The model under review builds one solid part; all positions refer to its coordinate system, in mm. A direction names the side the tool comes from. Coordinates: 2 decimals unless noted, no trailing zeros.
1) Machinability: for faces 1 (the flat face through (35, 0, 0)), 2 (the flat face through (43, 0, -14)), 3 (the conical face through (-40.1, 0.7, -13.8)), 4 (the flat face through (-39, 0, 10.75)), 5 (the flat face through (22, 0, -3.75)), which of the approach directions +Z, -Z, +X, -X, +Y, -Y give a long, thin tool a straight path to every point of the face, cutting with its end or side? Answer none if there is none.
2) Mouldability with a two-part tool opening along Z and no side actions: class faces 6 (the conical face through (-40.1, 0.7, 13.7)), 7 (the flat face through (-1, -1.5, 0)), 8 (the cylindrical face through (-42.61, -0.51, 14.21)) as released by +Z, released by -Z, zero draft, split by the parting line, or undercut.
3) Add section A-A, the plane y = -0.75. Give the number of separate pieces and of enclosed holes in the cut face, then the cut area to 3 significant figures.
4) For P1, Ø1.5, axis at y = -0.5, z = 9.5, coming from the -X side; P2, Ø0.9, axis at y = -0.5, z = -7.5, coming from the +X side, all flat-tipped, find the tip position at first contact; note any pin that passes through.
5) For line 1 (Z direction, x = 41.5, y = -0.8); line 2 (X direction, y = 0.8, z = -6); line 3 (Z direction, x = 37.5, y = 0.65), list the stretches that pass through material, from the lowest coordinate up.
from build123d import *

# Parameters (mm, degrees)
SKETCH1_W                                           = 86
SKETCH1_H                                           = 33.5
SKETCH1_W_2                                         = 20
SKETCH1_H_2                                         = 7
BOSS_EXTRUDE1_DEPTH                                 = 1.5
CSK_FOR_M3_COUNTERSUNK_FLAT_HEAD_SCREW1_D           = 3.4
CSK_FOR_M3_COUNTERSUNK_FLAT_HEAD_SCREW1_DEPTH       = 6
CSK_FOR_M3_COUNTERSUNK_FLAT_HEAD_SCREW1_CSINK_D     = 6.3
CSK_FOR_M3_COUNTERSUNK_FLAT_HEAD_SCREW1_CSINK_ANGLE = 90
CSK_FOR_M3_COUNTERSUNK_FLAT_HEAD_SCREW1_TIP         = 1.021463052
TAP_DRILL_FOR_M3_TAP1_D                             = 2.5
SKETCH13_W                                          = 3.5
SKETCH13_H                                          = 18
CUT_EXTRUDE3_DEPTH                                  = 48.943325917
CSK_FOR_M2_COUNTERSUNK_FLAT_HEAD_SCREW3_D           = 2.4
CSK_FOR_M2_COUNTERSUNK_FLAT_HEAD_SCREW3_DEPTH       = 4
CSK_FOR_M2_COUNTERSUNK_FLAT_HEAD_SCREW3_CSINK_D     = 4.4
CSK_FOR_M2_COUNTERSUNK_FLAT_HEAD_SCREW3_CSINK_ANGLE = 90
CSK_FOR_M2_COUNTERSUNK_FLAT_HEAD_SCREW3_TIP         = 0.721032743
SKETCH21_W                                          = 8
SKETCH21_H                                          = 21.5
CUT_EXTRUDE4_DEPTH                                  = 47.244594279
FILLET2_R                                           = 1


with BuildPart() as part:
    # Sketch1 → Boss-Extrude1 (new, symmetric)
    with BuildSketch(Plane(origin=(0, 0, 0), x_dir=(1, 0, 0), z_dir=(0, 1, 0))):
        Rectangle(SKETCH1_W, SKETCH1_H)
        with Locations((22.5, 7.25)):
            Rectangle(SKETCH1_W_2, SKETCH1_H_2, mode=Mode.SUBTRACT)
    extrude(amount=BOSS_EXTRUDE1_DEPTH, both=True)

    # CSK for M3 Countersunk Flat Head Screw1
    with Locations(Plane(origin=(0, 1.5, 0), x_dir=(1, 0, 0), z_dir=(0, 1, 0))):
        with Locations((-32, 8.93052757), (-32, -1.06947243)):
            CounterSinkHole(CSK_FOR_M3_COUNTERSUNK_FLAT_HEAD_SCREW1_D / 2, CSK_FOR_M3_COUNTERSUNK_FLAT_HEAD_SCREW1_CSINK_D / 2, depth=CSK_FOR_M3_COUNTERSUNK_FLAT_HEAD_SCREW1_DEPTH, counter_sink_angle=CSK_FOR_M3_COUNTERSUNK_FLAT_HEAD_SCREW1_CSINK_ANGLE)
            with Locations((0, 0, -(CSK_FOR_M3_COUNTERSUNK_FLAT_HEAD_SCREW1_DEPTH + CSK_FOR_M3_COUNTERSUNK_FLAT_HEAD_SCREW1_TIP / 2))):  # 118° drill point
                Cone(0, CSK_FOR_M3_COUNTERSUNK_FLAT_HEAD_SCREW1_D / 2, CSK_FOR_M3_COUNTERSUNK_FLAT_HEAD_SCREW1_TIP, mode=Mode.SUBTRACT)

    # Tap Drill for M3 Tap1 (through all)
    with Locations(Plane(origin=(0, 1.5, 0), x_dir=(1, 0, 0), z_dir=(0, 1, 0))):
        with Locations((-35, 12.75), (-35, -12.75), (35, -12.75), (35, 12.75)):
            Hole(TAP_DRILL_FOR_M3_TAP1_D / 2)

    # Sketch13 → Cut-Extrude3 (cut, through all)
    with BuildSketch(Plane.XZ.offset(11.5)):
        with Locations((-38.25, -0.25)):
            Rectangle(SKETCH13_W, SKETCH13_H)
    extrude(amount=-CUT_EXTRUDE3_DEPTH, mode=Mode.SUBTRACT)

    # CSK for M2 Countersunk Flat Head Screw3
    with Locations(Plane(origin=(0, 1.5, 0), x_dir=(1, 0, 0), z_dir=(0, 1, 0))):
        with Locations((-41.5, -13.75), (-41.5, 13.75), (41.5, 13.75), (41.5, -13.75)):
            CounterSinkHole(CSK_FOR_M2_COUNTERSUNK_FLAT_HEAD_SCREW3_D / 2, CSK_FOR_M2_COUNTERSUNK_FLAT_HEAD_SCREW3_CSINK_D / 2, depth=CSK_FOR_M2_COUNTERSUNK_FLAT_HEAD_SCREW3_DEPTH, counter_sink_angle=CSK_FOR_M2_COUNTERSUNK_FLAT_HEAD_SCREW3_CSINK_ANGLE)
            with Locations((0, 0, -(CSK_FOR_M2_COUNTERSUNK_FLAT_HEAD_SCREW3_DEPTH + CSK_FOR_M2_COUNTERSUNK_FLAT_HEAD_SCREW3_TIP / 2))):  # 118° drill point
                Cone(0, CSK_FOR_M2_COUNTERSUNK_FLAT_HEAD_SCREW3_D / 2, CSK_FOR_M2_COUNTERSUNK_FLAT_HEAD_SCREW3_TIP, mode=Mode.SUBTRACT)

    # Sketch21 → Cut-Extrude4 (cut, through all)
    with BuildSketch(Plane(origin=(0, 1.5, 0), x_dir=(1, 0, 0), z_dir=(0, 1, 0))):
        with Locations((-39, 0)):
            Rectangle(SKETCH21_W, SKETCH21_H)
        with Locations((39, 0)):
            Rectangle(SKETCH21_W, SKETCH21_H)
    extrude(amount=-CUT_EXTRUDE4_DEPTH, mode=Mode.SUBTRACT)

    # Fillet2
    fillet2_edges = [part.edges().sort_by_distance(p)[0] for p in [
        (35, 0, 10.75),
        (43, 0, 10.75),
        (43, 0, -10.75),
        (35, 0, -10.75),
        (-43, 0, 10.75),
        (-35, 0, 10.75),
        (-43, 0, -10.75),
        (-35, 0, -10.75),
        (12.5, 0, -3.75),
        (32.5, 0, -3.75),
        (32.5, 0, -10.75),
        (12.5, 0, -10.75),
    ]]
    fillet(fillet2_edges, radius=FILLET2_R)


solid = part.part
Geometry results:
1. face 1: +X, +Y, -Y
1. face 2: +Z, -Z, +X, +Y, -Y
1. face 3: +Y
1. face 4: -X, +Y, -Y
1. face 5: +Y, -Y
2. face 6: undercut
2. face 7: zero draft
2. face 8: undercut
3. separate pieces: 1
3. enclosed holes: 11
3. area: 2,340 mm2
4. P1: stops at x = -35.13
4. P2: stops at x = 35
5. line 1: z = -16.75 to -14.95, -12.55 to -10.75, 10.75 to 12.55, 14.95 to 16.75
5. line 2: x = -35 to 12.5, 32.5 to 35
5. line 3: z = -16.75 to -10.75, 10.75 to 16.75
